```python
from build123d import *

# Parameters (mm, degrees)
SKETCH1_W           = 39.920556732
SKETCH1_H           = 6.35
BOSS_EXTRUDE1_DEPTH = 6


with BuildPart() as part:
    # Sketch1 → Boss-Extrude1 (new body)
    with BuildSketch(Plane(origin=(0, 0, 2.54), x_dir=(-1, 0, 0), z_dir=(0, 0, -1))):
        Polygon((-48.535278366, 182.16527563), (-56.859833665, 182.455975506), (-56.859833665, 195.155975506), (-48.535278366, 195.446675383), (-48.535278366, 204.971675383), (-29.485278366, 204.971675383), (-29.485278366, 239.9538), (29.485278366, 239.9538), (29.485278366, 204.971675383), (48.535278366, 204.971675383), (48.535278366, 195.446675383), (56.859833665, 195.155975506), (56.859833665, 182.455975506), (48.535278366, 182.16527563), (48.535278366, 172.64027563), (-48.535278366, 172.64027563), align=None)
        with Locations((0, 228.6)):
            Rectangle(SKETCH1_W, SKETCH1_H, mode=Mode.SUBTRACT)
    extrude(amount=-BOSS_EXTRUDE1_DEPTH)


solid = part.part
```
Input: part model. Units: mm. Frame: model coordinates. A direction names the side the tool comes from. Coordinates: 2 decimals unless noted, no trailing zeros. Loops run counter-clockwise (first coordinate to the right, second up) from the corner with the lowest first, then second, coordinate; pieces in that order, holes last. Notation, with made-up numbers: (4.25, 28.25) - (20.25, 28.25) arc R22 cw to (20.25, 46.25) - close; hole circle Ø11 at (-4, 73). An arc over 180 degrees is marked (long way). Answer in a Markdown table with one row per item.
(1) Set-up query: faces 5 (the face through (-39, 204.972, 5)), 6 (the face through (-48.535, 177, 5)), 7 (the face through (48.535, 200, 5)), 8 (the face through (48.535, 177, 5)). Return all of +Z, -Z, +X, -X, +Y, -Y with unobstructed straight access to the full face (end or side cutting, diameter ignored); none if empty.
Model answer:
| item | result |
|---|---|
| face 5 | +Z, -Z, -X, +Y |
| face 6 | +Z, -Z, -X, -Y |
| face 7 | +Z, -Z, +X, +Y |
| face 8 | +Z, -Z, +X, -Y |
(2) Cut plane B-B on x = -5. Output: boundary loops of the cut face in (y, z) (3 decimals).
Model answer:
| item | result |
|---|---|
| outline | (172.64, 2.54) - (225.425, 2.54) - (225.425, 8.54) - (172.64, 8.54) - close; (231.775, 2.54) - (239.954, 2.54) - (239.954, 8.54) - (231.775, 8.54) - close |
(3) Material intervals for L1, parallel to Y at x = 1.5, z = 4.75 (3 decimals); L2, parallel to X at y = 229.5, z = 6.2; L3, parallel to Y at x = 34, z = 6.6, sorted ascending. Write a range as from..to.
Model answer:
| item | result |
|---|---|
| L1 | y = 172.64..225.425, 231.775..239.954 |
| L2 | x = -29.49..-19.96, 19.96..29.49 |
| L3 | y = 172.64..204.97 |
(4) Cut plane A-A on y = 226.5. Output: boundary loops of the cut face in (x, z).
Model answer:
| item | result |
|---|---|
| outline | (-29.49, 2.54) - (-19.96, 2.54) - (-19.96, 8.54) - (-29.49, 8.54) - close; (19.96, 2.54) - (29.49, 2.54) - (29.49, 8.54) - (19.96, 8.54) - close |
(5) Mould query, pull axis X, two halves, no side actions, for faces 1 (the face through (-19.96, 229, 5)), 2 (the face through (-48.535, 200, 5)), 3 (the face through (-1, 199, 8.54)), 4 (the face through (0, 225.425, 5)). Classes: pulls with the +X half, pulls with the -X half, needs draft (parallel to the pull), parting line crosses it, or undercut.
Model answer:
| item | result |
|---|---|
| face 1 | undercut |
| face 2 | pulls with the -X half |
| face 3 | needs draft |
| face 4 | undercut |
(6) Cut plane D-D on y = 212. Output: boundary loops of the cut face in (x, z).
Model answer:
| item | result |
|---|---|
| outline | (-29.49, 2.54) - (29.49, 2.54) - (29.49, 8.54) - (-29.49, 8.54) - close |
(7) Pin query (flat end, axial travel): P1, Ø1.8, axis at y = 176.5, z = 6.5, coming from the -X side; P2, Ø1.8, axis at y = 216.5, z = 6.5, coming from the -X side; P3, Ø2, axis at y = 196.5, z = 5, coming from the +X side. Return the tip coordinate at first contact, or that it passes through.
Model answer:
| item | result |
|---|---|
| P1 | stops at x = -48.54 |
| P2 | stops at x = -29.49 |
| P3 | stops at x = 48.54 |
(8) Cut plane C-C on z = 4.55. Output: boundary loops of the cut face in (x, y) (3 decimals), plus the area to 3 significant figures.
Model answer:
| item | result |
|---|---|
| outline | (-56.86, 182.456) - (-48.535, 182.165) - (-48.535, 172.64) - (48.535, 172.64) - (48.535, 182.165) - (56.86, 182.456) - (56.86, 195.156) - (48.535, 195.447) - (48.535, 204.972) - (29.485, 204.972) - (29.485, 239.954) - (-29.485, 239.954) - (-29.485, 204.972) - (-48.535, 204.972) - (-48.535, 195.447) - (-56.86, 195.156) - close; hole (-19.96, 225.425) - (19.96, 225.425) - (19.96, 231.775) - (-19.96, 231.775) - close |
| area | 5,160 mm² |
